Model file for the job. Use its own axes, mm. Coordinates: 2 decimals unless noted, no trailing zeros. Order: outer loops, then holes, each group sorted by start corner. A loop starts at its lowest first (then second) coordinate and runs counter-clockwise, first axis right, second up. Notation, with made-up numbers: (50.5, 17) -> (100.5, 17) arc R4 cw to (100.5, 24) -> close; hole circle Ø4 at (87, 83.25). An arc over 180 degrees is marked (long way). Return JSON: item names as keys, results as strings. Group by question number.
1) Cut at B-B (x = -1.05). State how many separate pieces and enclosed holes the cut face has, and give its area (3 significant figures).
2) Probe line 1 (Z direction, x = -0.7, y = 27.5); line 2 (Y direction, x = -1.7, z = 67.38); line 3 (Z direction, x = -2.7, y = 33). List the from-to ranges inside material, lowest first.
3) Pull direction Z, two halves, no side cores. Call faces 1 (the flat face through (0, 2, 2)), 2 (the cylindrical face through (-1.52, -18.32, 56.39)): +Z half, -Z half, draft (parallel to the pull), parting line (faces both ways), or undercut.
4) Cut at A-A (y = -18.8). Write the cut outline in (x, z).
5) Flat gauge pins, fed straight in: pin 1 (0.9 mm diameter, centred on x = -1.5, z = -53.5, fed in from +Y); pin 2 (1.5 mm diameter, centred on x = -2, y = 39.5, fed in from -Z); pin 3 (0.9 mm diameter, centred on x = -1.5, y = 40, fed in from +Z). Where does each tip first touch, or does it go through?
6) Cut at C-C (z = 35.5). Write the cut outline in (x, y), and give its area (3 significant figures).
from build123d import *

# Parameters (mm, degrees)
SKETCH1_W               = 279.4
SKETCH1_H               = 76.2
BOSS_EXTRUDE1_DEPTH     = 3
SKETCH3_W               = 3
SKETCH3_H               = 15
CUT_EXTRUDE1_DEPTH      = 145.833352512
LPATTERN1_COUNT         = 3
LPATTERN1_PITCH         = 22.8
MIRROR1_COPY_1_SKETCH_W = 3
MIRROR1_COPY_1_SKETCH_H = 15
MIRROR1_COPY_1_DEPTH    = 145.833352512
MIRROR1_COPY_2_SKETCH_W = 3
MIRROR1_COPY_2_SKETCH_H = 15
MIRROR1_COPY_2_DEPTH    = 145.833352512
SKETCH6_W               = 3
SKETCH6_H               = 7.8
CUT_EXTRUDE2_DEPTH      = 145.833352512
LPATTERN2_COUNT         = 4
LPATTERN2_PITCH         = 22.8
SKETCH8_W               = 3
SKETCH8_H               = 7.8
BOSS_EXTRUDE2_DEPTH     = 3
LPATTERN4_COUNT         = 11
LPATTERN4_PITCH         = 22.8
SKETCH9_R               = 11
CUT_EXTRUDE3_DEPTH      = 146.651295909


with BuildPart() as part:
    # Sketch1 → Boss-Extrude1 (new body)
    with BuildSketch(Plane(origin=(0, 0, 0), x_dir=(0, 0, -1), z_dir=(1, 0, 0))):
        Rectangle(SKETCH1_W, SKETCH1_H)
    extrude(amount=-BOSS_EXTRUDE1_DEPTH)

    # Sketch3 → Cut-Extrude1 (cut, through all)
    with BuildSketch(Plane.ZY.offset(3)):
        with Locations((133.2, 22.8)):
            Rectangle(SKETCH3_W, SKETCH3_H)
    cut_extrude1 = extrude(amount=-CUT_EXTRUDE1_DEPTH, mode=Mode.SUBTRACT)

    # LPattern1: Cut-Extrude1 ×3
    with Locations(*[(0, -i * LPATTERN1_PITCH, 0) for i in range(1, LPATTERN1_COUNT)]):
        add(cut_extrude1, mode=Mode.SUBTRACT)

    # Mirror1: Cut-Extrude1 across plane
    add(cut_extrude1.mirror(Plane.XY), mode=Mode.SUBTRACT)

    # Mirror1 copy 1 sketch → Mirror1 copy 1 (cut, through all)
    with BuildSketch(Plane(origin=(-3, -22.8, 0), x_dir=(0, 0, -1), z_dir=(-1, 0, 0))):
        with Locations((133.2, -22.8)):
            Rectangle(MIRROR1_COPY_1_SKETCH_W, MIRROR1_COPY_1_SKETCH_H)
    extrude(amount=-MIRROR1_COPY_1_DEPTH, mode=Mode.SUBTRACT)

    # Mirror1 copy 2 sketch → Mirror1 copy 2 (cut, through all)
    with BuildSketch(Plane(origin=(-3, -45.6, 0), x_dir=(0, 0, -1), z_dir=(-1, 0, 0))):
        with Locations((133.2, -22.8)):
            Rectangle(MIRROR1_COPY_2_SKETCH_W, MIRROR1_COPY_2_SKETCH_H)
    extrude(amount=-MIRROR1_COPY_2_DEPTH, mode=Mode.SUBTRACT)

    # Sketch6 → Cut-Extrude2 (cut, through all)
    with BuildSketch(Plane.ZY.offset(3)):
        with Locations((1.56, 34.2)):
            Rectangle(SKETCH6_W, SKETCH6_H)
    cut_extrude2 = extrude(amount=-CUT_EXTRUDE2_DEPTH, mode=Mode.SUBTRACT)

    # LPattern2: Cut-Extrude2 ×4
    with Locations(*[(0, -i * LPATTERN2_PITCH, 0) for i in range(1, LPATTERN2_COUNT)]):
        add(cut_extrude2, mode=Mode.SUBTRACT)

    # Sketch8 → Boss-Extrude2 (add)
    with BuildSketch(Plane(origin=(0, 38.1, 0), x_dir=(1, 0, 0), z_dir=(0, 1, 0))):
        with Locations((-1.5, 113)):
            Rectangle(SKETCH8_W, SKETCH8_H)
    boss_extrude2 = extrude(amount=BOSS_EXTRUDE2_DEPTH)

    # LPattern4: Boss-Extrude2 ×11, 1 skipped
    with Locations(*[(0, 0, i * LPATTERN4_PITCH) for i in range(1, LPATTERN4_COUNT) if i not in (5,)]):
        add(boss_extrude2)

    # Sketch9 → Cut-Extrude3 (cut, through all)
    with BuildSketch(Plane.ZY.offset(3)):
        with Locations((67.38, -18.8)):
            Circle(SKETCH9_R)
    extrude(amount=-CUT_EXTRUDE3_DEPTH, mode=Mode.SUBTRACT)


solid = part.part
Answers below:
{
 "1": {"separate pieces": "1", "enclosed holes": "9", "area": "20,800 mm^2"},
 "2": {"line 1": "z = -139.7 to -134.7, -131.7 to 131.7, 134.7 to 139.7", "line 2": "y = -38.1 to -29.8, -7.8 to 41.1", "line 3": "z = -139.7 to 0.06, 3.06 to 139.7"},
 "3": {"face 1": "draft", "face 2": "undercut"},
 "4": {"outline": "(-3, -139.7) -> (0, -139.7) -> (0, -134.7) -> (-3, -134.7) -> close; (-3, -131.7) -> (0, -131.7) -> (0, 56.38) -> (-3, 56.38) -> close; (-3, 78.38) -> (0, 78.38) -> (0, 131.7) -> (-3, 131.7) -> close; (-3, 134.7) -> (0, 134.7) -> (0, 139.7) -> (-3, 139.7) -> close"},
 "5": {"pin 1": "stops at y = 38.1", "pin 2": "stops at z = -116.9", "pin 3": "stops at z = 118.9"},
 "6": {"outline": "(-3, -38.1) -> (0, -38.1) -> (0, 38.1) -> (-3, 38.1) -> close", "area": "229 mm^2"}
}
